```python
from build123d import *

# Parameters (mm, degrees)
FILLET1_R = 3.175


with BuildPart() as part:
    # Sketch1 → Revolve2 (revolve)
    with BuildSketch(Plane.XY):
        with BuildLine():
            Line((-25.4, -6.141632853), (-25.4, 3.383367147))
            Line((-25.4, 3.383367147), (-19.05, 3.383367147))
            Line((-19.05, 3.383367147), (-19.05, 95.458367147))
            ThreePointArc((-19.05, 95.458367147), (-14.517976471, 111.753635849), (-2.223442899, 123.369119633))
            ThreePointArc((-2.223442899, 123.369119633), (-1.145335288, 123.78023171), (0, 123.9200038))
            Line((0, 123.9200038), (0, 95.458367147))
            Line((0, 95.458367147), (0, 0))
            Line((0, 0), (0, -56.941632853))
            Line((0, -56.941632853), (-19.05, -56.941632853))
            Line((-19.05, -56.941632853), (-19.05, -6.141632853))
            Line((-19.05, -6.141632853), (-25.4, -6.141632853))
        make_face()
    revolve(axis=Axis((0, 95.458367147, 0), (0, -1, 0)))

    # Fillet1
    fillet1_edges = [part.edges().sort_by_distance(p)[0] for p in [
        (19.05, 3.383367147, 0),
        (19.05, -6.141632853, 0),
    ]]
    fillet(fillet1_edges, radius=FILLET1_R)


solid = part.part
```
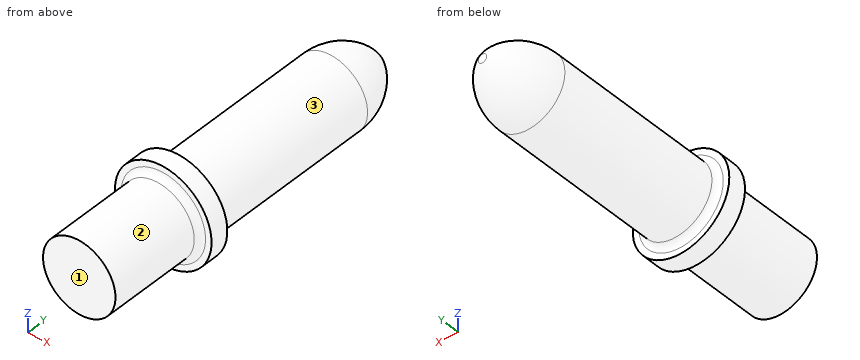
Input: part model. Units: mm. Frame: model coordinates. Face numbers are marked on the shaded views. A direction names the side the tool comes from. Give positions to 0.01 mm unless a question says otherwise; leave off trailing zeros. Loops run counter-clockwise (first coordinate to the right, second up) from the corner with the lowest first, then second, coordinate; pieces in that order, holes last. Notation, with made-up numbers: (22.5, 47) -> (56.5, 47) arc R24 cw to (56.5, 62) -> close; hole circle Ø7 at (24.5, 63). An arc over 180 degrees is marked (long way). Use a Markdown table: item, result.
Q1. Ray query, probe 1 along Y at (x, z) = (19, 14.5); probe 2 along Z at (x, y) = (-3, -29); probe 3 along Z at (x, y) = (-4, 54). Return the intervals inside material, ascending. Write a range as from..to.
Entries:
| item | result |
|---|---|
| probe 1 | y = -6.14..3.38 |
| probe 2 | z = -18.81..18.81 |
| probe 3 | z = -18.63..18.63 |
Q2. First-contact query: P1, Ø4, axis at y = 46, z = 0, coming from the -X side; P2, Ø10, axis at x = -15.5, y = 51.5, coming from the +Z side; P3, Ø10, axis at y = -4, z = -9, coming from the +X side. Flat tips, straight axial feed; report the tip coordinate or a pass-through.
Entries:
| item | result |
|---|---|
| P1 | stops at x = -19.05 |
| P2 | stops at z = 15.9 |
| P3 | stops at x = 25.08 |
Q3. Access query for the marked faces 1, 2 and 3. Directions: +Z, -Z, +X, -X, +Y, -Y. A direction counts if a zero-diameter tool reaches every point of the face in a straight line with its end or side. Return the directions, or none.
Entries:
| item | result |
|---|---|
| face 1 | +Z, -Z, +X, -X, -Y |
| face 2 | -Y |
| face 3 | +Y |
Q4. Section query B-B, the plane y = 42.5. Return the cut outline in (x, z).
Entries:
| item | result |
|---|---|
| outline | circle Ø38.1 at (0, 0) |
Q5. Section query A-A, the plane y = -4. Return the cut outline in (x, z), plus the area to 3 significant figures.
Entries:
| item | result |
|---|---|
| outline | circle Ø50.8 at (0, 0) |
| area | 2,030 mm² |
